CAD build for the part. Positions are in the model's coordinates, mm. Face numbers are marked on the shaded views. A direction names the side the tool comes from. Coordinates: 2 decimals unless noted, no trailing zeros. Loops run counter-clockwise (first coordinate to the right, second up) from the corner with the lowest first, then second, coordinate; pieces in that order, holes last.
1) Pin check, flat tips, straight feed: pin 1 Ø5 at (x, y) = (107.5, 14.5) entering from +Z; pin 2 Ø0.5 at (y, z) = (53, 4.5) entering from -X; pin 3 Ø6.5 at (x, y) = (107.5, 52.5) entering from -Z; pin 4 Ø5 at (y, z) = (27.5, 4.5) entering from -X. Stop position of each tip, or through.
2) Saw through at B-B, the plane z = 4.75. Write the cut outline in (x, y).
3) Saw through at C-C, the plane y = 37. Write the cut outline in (x, z), and give its area (3 significant figures).
4) Which spindle directions (+Z, -Z, +X, -X, +Y, -Y) get a long thin tool onto all of the face, cutting with end or side? Do the marked faces 1, 2, 3, 4 and 5. Say none if no direction does.
5) Wall check: line 1 along X through (y, z) = (17, 4.75); line 2 along Y through (x, z) = (108, 3.75); line 3 along X through (y, z) = (19.5, 7.75). Give the ranges that are in metal, low to high.
6) Saw through at A-A, the plane y = 15.5. Write the cut outline in (x, z).
7) Saw through at D-D, the plane x = 108.5. Write the cut outline in (y, z), and give its area (3 significant figures).
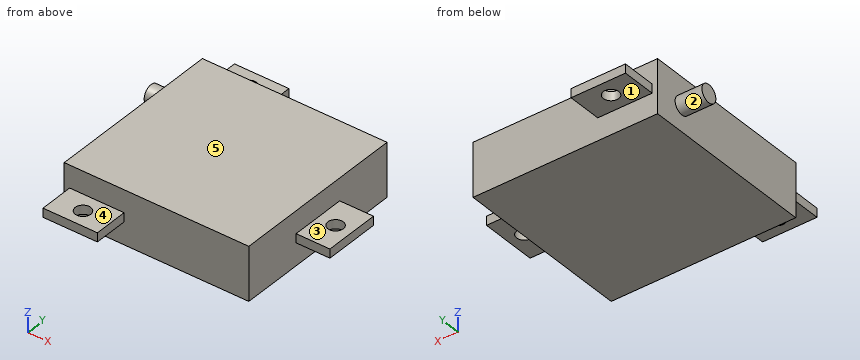
```python
from build123d import *

# Parameters (mm, degrees)
SKETCH1_W           = 32.7406
SKETCH1_H           = 31.5722
BOSS_EXTRUDE1_DEPTH = 3.9624
SKETCH2_R           = 1.3716
BOSS_EXTRUDE2_DEPTH = 1.5875
SKETCH3_W           = 32.7406
SKETCH3_H           = 31.5722
BOSS_EXTRUDE3_DEPTH = 3.9624
SKETCH4_R           = 1.5875
BOSS_EXTRUDE4_DEPTH = 4.7625


with BuildPart() as part:
    # Sketch1 → Boss-Extrude1 (new body)
    with BuildSketch(Plane.XY):
        with Locations((116.543894781, 33.611845874)):
            Rectangle(SKETCH1_W, SKETCH1_H)
    extrude(amount=BOSS_EXTRUDE1_DEPTH)

    # Sketch2 → Boss-Extrude2 (add)
    with BuildSketch(Plane.XY.offset(3.9624)):
        Polygon((100.173594781, 49.397945874), (101.138794781, 49.397945874), (101.138794781, 55.493945874), (110.790794781, 55.493945874), (110.790794781, 49.397945874), (132.914194781, 49.397945874), (132.914194781, 38.590245874), (138.908594781, 38.590245874), (138.908594781, 28.633445874), (132.914194781, 28.633445874), (132.914194781, 17.825745874), (110.790794781, 17.825745874), (110.790794781, 11.729745874), (101.138794781, 11.729745874), (101.138794781, 17.825745874), (100.173594781, 17.825745874), align=None)
        with Locations((136.050967198, 33.611845874)):
            Circle(SKETCH2_R, mode=Mode.SUBTRACT)
        with Locations((105.964794781, 52.572945874)):
            Circle(SKETCH2_R, mode=Mode.SUBTRACT)
        with Locations((105.964794781, 14.650745874)):
            Circle(SKETCH2_R, mode=Mode.SUBTRACT)
    extrude(amount=BOSS_EXTRUDE2_DEPTH)

    # Sketch3 → Boss-Extrude3 (add)
    with BuildSketch(Plane.XY.offset(5.5499)):
        with Locations((116.543894781, 33.611845874)):
            Rectangle(SKETCH3_W, SKETCH3_H)
    extrude(amount=BOSS_EXTRUDE3_DEPTH)

    # Sketch4 → Boss-Extrude4 (add)
    with BuildSketch(Plane.ZY.offset(-100.173594781)):
        with Locations(Location((4.52755, 43.809945874, 0), (0, 0, 180))):
            Circle(SKETCH4_R)
    extrude(amount=BOSS_EXTRUDE4_DEPTH)


solid = part.part
```
Data:
1. pin 1: stops at z = 5.55
1. pin 2: stops at x = 101.14
1. pin 3: stops at z = 0
1. pin 4: stops at x = 100.17
2. outline: (95.41, 42.24) - (100.17, 42.24) - (100.17, 17.83) - (101.14, 17.83) - (101.14, 11.73) - (110.79, 11.73) - (110.79, 17.83) - (132.91, 17.83) - (132.91, 28.63) - (138.91, 28.63) - (138.91, 38.59) - (132.91, 38.59) - (132.91, 49.4) - (110.79, 49.4) - (110.79, 55.49) - (101.14, 55.49) - (101.14, 49.4) - (100.17, 49.4) - (100.17, 45.38) - (95.41, 45.38) - close; hole circle Ø2.74 at (105.96, 14.65); hole circle Ø2.74 at (105.96, 52.57); hole circle Ø2.74 at (136.05, 33.61)
3. outline: (100.17, 0) - (132.91, 0) - (132.91, 3.96) - (138.91, 3.96) - (138.91, 5.55) - (132.91, 5.55) - (132.91, 9.51) - (100.17, 9.51) - close
3. area: 321 mm2
4. face 1: -Z, +X, -X, +Y
4. face 2: -X
4. face 3: +Z, +X, +Y, -Y
4. face 4: +Z, +X, -X, -Y
4. face 5: +Z, +X, -X, +Y, -Y
5. line 1: x = 101.14 to 110.79
5. line 2: y = 17.83 to 49.4
5. line 3: x = 100.17 to 132.91
6. outline: (101.14, 3.96) - (104.89, 3.96) - (104.89, 5.55) - (101.14, 5.55) - close; (107.04, 3.96) - (110.79, 3.96) - (110.79, 5.55) - (107.04, 5.55) - close
7. outline: (11.73, 3.96) - (17.83, 3.96) - (17.83, 0) - (49.4, 0) - (49.4, 3.96) - (55.49, 3.96) - (55.49, 5.55) - (49.4, 5.55) - (49.4, 9.51) - (17.83, 9.51) - (17.83, 5.55) - (11.73, 5.55) - close
7. area: 320 mm2
